The listing builds one solid part. Answer for the finished solid, in the listing's coordinates (mm). A direction names the side the tool comes from. Round coordinates to 2 decimals unless told otherwise and drop trailing zeros. Order: outer loops, then holes, each group sorted by start corner. A loop starts at its lowest first (then second) coordinate and runs counter-clockwise, first axis right, second up. Notation, with made-up numbers: (39.25, 89) -> (58.25, 89) arc R22 cw to (58.25, 110) -> close; hole circle Ø5 at (36, -30). An arc over 180 degrees is marked (long way). Return JSON: item names as keys, results as strings. Group by question number.
(1) The part is cut by section A-A (z = 0). Determine the outline of the cut face in (x, y).
(2) Consider line 1 (X direction, y = 1.3, z = 0); line 2 (Y direction, x = 4, z = -1.5); line 3 (Z direction, x = 15, y = 3.85). Determine where each line is inside the solid, lowest interval first. Write a range as [from, to].
(3) Each of these flat-tipped pins is pushed along its axis until it touches: pin 1 (1 mm diameter, centred on y = 2, z = 6, fed in from +X); pin 2 (3.5 mm diameter, centred on x = 30, z = 0, fed in from -Y); pin 3 (1 mm diameter, centred on y = 0.5, z = -7, fed in from +X). Where does it stop, or does it pass through?
(4) The part is cut by section D-D (y = 2.6). Determine the outline of the cut face in (x, z).
(5) The part is cut by section B-B (x = 15). Determine the outline of the cut face in (y, z), plus the area to 4 significant figures.
(6) Determine the mould class of faces 3 (the face through (28, 1, 0)), 4 (the face through (12, 4.5, 5)), 5 (the face through (15, 3, 6)), 6 (the face through (-10, 1, 0)) for opening direction X: +X half, -X half, draft (parallel to the pull), parting line (faces both ways), or undercut.
(7) Which of the six approach directions +Z, -Z, +X, -X, +Y, -Y give full straight-line access (tool end or side, diameter ignored) to faces 1 (the face through (15, 1, -10)), 2 (the face through (15, 2, 0))?
(8) The part is cut by section C-C (y = 0.55). Determine the outline of the cut face in (x, z).
from build123d import *

# Parameters (mm, degrees)
EXTRUDE_1_DEPTH     = 2
SKETCH_2_R          = 2
CUT_EXTRUDE_1_DEPTH = 2
SKETCH_3_R          = 6
SKETCH_3_R_2        = 5.5
EXTRUDE_2_DEPTH     = 2.5
CUT_EXTRUDE_2_DEPTH = 2.5


with BuildPart() as part:
    # 草图1 → 凸台-拉伸1 (new body)
    with BuildSketch(Plane(origin=(0, 0, 0), x_dir=(1, 0, 0), z_dir=(0, 1, 0))):
        with BuildLine():
            Line((0, 10), (30, 10))
            ThreePointArc((30, 10), (40, 0), (30, -10))
            Line((30, -10), (0, -10))
            ThreePointArc((0, -10), (-10, 0), (0, 10))
        make_face()
    extrude(amount=EXTRUDE_1_DEPTH)

    # 草图2 → 切除-拉伸1 (cut)
    with BuildSketch(Plane(origin=(0, 2, 0), x_dir=(1, 0, 0), z_dir=(0, 1, 0))):
        with Locations(Location((0, 0, 0), (0, 0, 270))):
            Circle(SKETCH_2_R)
        with Locations(Location((30, 0, 0), (0, 0, 270))):
            Circle(SKETCH_2_R)
    extrude(amount=-CUT_EXTRUDE_1_DEPTH, mode=Mode.SUBTRACT)

    # 草图3 → 凸台-拉伸2 (add)
    with BuildSketch(Plane(origin=(0, 2, 0), x_dir=(1, 0, 0), z_dir=(0, 1, 0))):
        with Locations(Location((15, 0, 0), (0, 0, 270))):
            Circle(SKETCH_3_R)
        with Locations(Location((15, 0, 0), (0, 0, 270))):
            Circle(SKETCH_3_R_2, mode=Mode.SUBTRACT)
    extrude(amount=EXTRUDE_2_DEPTH)

    # 草图4 → 切除-拉伸2 (cut)
    with BuildSketch(Plane(origin=(0, 2, 0), x_dir=(1, 0, 0), z_dir=(0, 1, 0))):
        with BuildLine():
            Line((15, 0), (13, 5.656854249))
            ThreePointArc((13, 5.656854249), (15, 6), (17, 5.656854249))
            Line((17, 5.656854249), (15, 0))
        make_face()
    extrude(amount=CUT_EXTRUDE_2_DEPTH, mode=Mode.SUBTRACT)


solid = part.part
Answer below:
{
 "1": {"outline": "(-10, 0) -> (-2, 0) -> (-2, 2) -> (-10, 2) -> close; (2, 0) -> (28, 0) -> (28, 2) -> (21, 2) -> (21, 4.5) -> (20.5, 4.5) -> (20.5, 2) -> (9.5, 2) -> (9.5, 4.5) -> (9, 4.5) -> (9, 2) -> (2, 2) -> close; (32, 0) -> (40, 0) -> (40, 2) -> (32, 2) -> close"},
 "2": {"line 1": "x = [-10, -2], [2, 28], [32, 40]", "line 2": "y = [0, 2]", "line 3": "z = [5.5, 6]"},
 "3": {"pin 1": "stops at x = 38.35", "pin 2": "passes through", "pin 3": "stops at x = 37.6"},
 "4": {"outline": "(13, -5.66) -> (13.17, -5.19) arc R5.5 cw (long way) to (16.83, -5.19) -> (17, -5.66) arc R6 ccw (long way) to start"},
 "5": {"outline": "(0, -10) -> (2, -10) -> (2, 5.5) -> (4.5, 5.5) -> (4.5, 6) -> (2, 6) -> (2, 10) -> (0, 10) -> close", "area": "41.25 mm²"},
 "6": {"face 3": "undercut", "face 4": "draft", "face 5": "parting line", "face 6": "-X half"},
 "7": {"face 1": "-Z, +X, -X, +Y, -Y", "face 2": "+Y"},
 "8": {"outline": "(0, -10) -> (30, -10) arc R10 ccw to (30, 10) -> (0, 10) arc R10 ccw to start; hole circle Ø4 at (0, 0); hole circle Ø4 at (30, 0)"}
}
